Check sheet for the modelled part. Datum: model origin and axes. Units: mm. Face numbers are marked on the shaded views. A direction names the side the tool comes from. Round coordinates to 2 decimals unless told otherwise and drop trailing zeros. Write each loop counter-clockwise with the first axis right and the second up, starting at its lowest first coordinate (ties: lowest second). Pieces come first, ordered by that corner, then holes.
Item 1: Cross-section at C-C on z = 1.5. Enter the section's corners in (x, y), plus the area to 3 significant figures.
Item 2: Cross-section at B-B on y = -11.5. Enter the section's corners in (x, z), plus the area to 3 significant figures.
Item 3: Cross-section at D-D on x = -111.5. Enter the section's corners in (y, z).
Item 4: Tool access check on the marked faces 1 and 2. Record the directions out of +Z, -Z, +X, -X, +Y, -Y that give a thin tool (end or side, any length) a straight path to the whole face; none if there is none.
Item 5: Material ranges on line 1 (Y direction, x = -42, z = 3.5); line 2 (Y direction, x = 147.5, z = 1.25); line 3 (Z direction, x = -74, y = 6), recorded low to high.
Item 6: Go/stop test with flat-tipped pins: pin 1 Ø1.5 at (y, z) = (12, 8.5) entering from -X; pin 2 Ø5 at (x, z) = (151.85, 5.24) entering from +Y; pin 3 Ø0.9 at (y, z) = (-5, 2) entering from +X; pin 4 Ø4 at (y, z) = (0, 3.5) entering from +X. Record where each tip stops, or that it passes through.
Item 7: Cross-section at A-A on x = 101. Enter the section's corners in (y, z).
from build123d import *

# Parameters (mm, degrees)
F1_DEPTH = 5
F2_W     = 25
F2_H     = 8
F3_DEPTH = 5
F4_R     = 1.5
F5_DEPTH = 30.3


with BuildPart() as f1:
    # F0 (on Top) → F1 (new body)
    with BuildSketch(Plane.XY):
        with BuildLine():
            Line((-153.607063, -15), (163.607063, -15))
            Line((163.607063, -15), (163.607063, -7))
            Line((163.607063, -7), (-66.559589, -7))
            Line((-66.559589, -7), (-66.559589, -4))
            Line((-66.559589, -4), (138.750769, -4))
            Line((138.750769, -4), (138.750769, 4))
            Line((138.750769, 4), (-66.559589, 4))
            Line((-66.559589, 4), (-66.559589, 7))
            Line((-66.559589, 7), (163.607063, 7))
            Line((163.607063, 7), (163.607063, 15))
            Line((163.607063, 15), (-153.607063, 15))
            ThreePointArc((-153.607063, 15), (-160.678131, 12.071068), (-163.607063, 5))
            Line((-163.607063, 5), (-163.607063, -5))
            ThreePointArc((-163.607063, -5), (-160.678131, -12.071068), (-153.607063, -15))
        make_face()
    extrude(amount=F1_DEPTH)

    # F2 (on face) → F3 (join)
    with BuildSketch(Plane.XY.offset(5)):
        with Locations((151.107063, -11)):
            Rectangle(F2_W, F2_H)
        with Locations((151.107063, 11)):
            Rectangle(F2_W, F2_H)
    extrude(amount=F3_DEPTH)

    # F4 (on face) → F5 (cut)
    with BuildSketch(Plane.XZ.offset(15)):
        with Locations((151.84553, 5.24334)):
            Circle(F4_R)
    extrude(amount=-F5_DEPTH, mode=Mode.SUBTRACT)


solid = f1.part
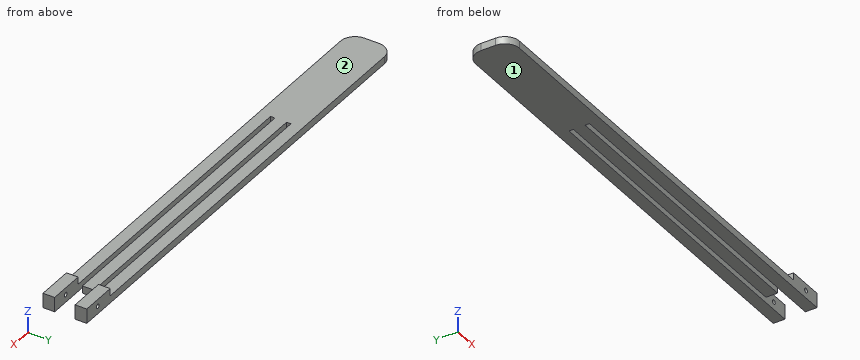
Response values:
1. outline: (-163.61, -5) arc R10 ccw to (-153.61, -15) - (163.61, -15) - (163.61, -7) - (-66.56, -7) - (-66.56, -4) - (138.75, -4) - (138.75, 4) - (-66.56, 4) - (-66.56, 7) - (163.61, 7) - (163.61, 15) - (-153.61, 15) arc R10 ccw to (-163.61, 5) - close
1. area: 8,190 mm2
2. outline: (-161.21, 0) - (163.61, 0) - (163.61, 10) - (138.61, 10) - (138.61, 5) - (-161.21, 5) - close; hole circle Ø3 at (151.85, 5.24)
2. area: 1,740 mm2
3. outline: (-15, 0) - (15, 0) - (15, 5) - (-15, 5) - close
4. face 1: -Z, +X, -X, +Y, -Y
4. face 2: +Z, -X, +Y, -Y
5. line 1: y = -15 to -7, -4 to 4, 7 to 15
5. line 2: y = -15 to -7, 7 to 15
5. line 3: z = 0 to 5
6. pin 1: stops at x = 138.61
6. pin 2: stops at y = 15
6. pin 3: stops at x = -66.56
6. pin 4: stops at x = 138.75
7. outline: (-15, 0) - (-7, 0) - (-7, 5) - (-15, 5) - close; (-4, 0) - (4, 0) - (4, 5) - (-4, 5) - close; (7, 0) - (15, 0) - (15, 5) - (7, 5) - close
